CAD build for the part. Positions are in the model's coordinates, mm. A direction names the side the tool comes from. Give positions to 0.01 mm unless a question says otherwise; leave off trailing zeros. Loops run counter-clockwise (first coordinate to the right, second up) from the corner with the lowest first, then second, coordinate; pieces in that order, holes last.
Item 1: Mould opens along Z. For faces 4 (the flat face through (0, 0, -8)), 5 (the cylindrical face through (4.46, 0.59, -0.25)), 6 (the cylindrical face through (5, 1.6, 6.2)), 7 (the flat face through (0, 0, 9.76)) say: released by +Z, released by -Z, zero draft, split by the parting line, or undercut.
Item 2: Saw through at D-D on z = -2. Give the cut face in (x, y), plus the area to 3 significant figures.
Item 3: Which spindle directions (+Z, -Z, +X, -X, +Y, -Y) get a long thin tool onto all of the face, cutting with end or side? Do faces 1 (the cylindrical face through (-1.91, -8.62, 1.36)), 2 (the cylindrical face through (4.46, 0.59, -7.51)), 3 (the flat face through (4, -4, 2.76)). Say none if no direction does.
Item 4: Drop flat-ended pins along their axis: P1, Ø1, axis at x = 2.5, z = 0, coming from the +Y side; P2, Ø8, axis at y = -3.5, z = -5.5, coming from the -X side; P3, Ø4, axis at y = -4, z = 3, coming from the +X side. Give the stop position or say it passes through.
Item 5: Saw through at C-C on z = 1.5. Give the cut face in (x, y), plus the area to 3 significant figures.
Item 6: Probe probe 1 along Z at (x, y) = (4.5, -4.5); probe 2 along Z at (x, y) = (3, -4.25); probe 3 along X at (y, z) = (-1.5, -3). List the from-to ranges inside material, lowest first.
from build123d import *

# Parameters (mm, degrees)
F0_R     = 8.83
F1_DEPTH = 2.76
F4_R     = 5.25
F5_DEPTH = 7


with BuildPart() as f1:
    # F0 (on Top) → F1 (new body)
    with BuildSketch(Plane.XY):
        Circle(F0_R)
    extrude(amount=F1_DEPTH)

    # F2 (on Right) → F3 (revolve)
    with BuildSketch(Plane.YZ):
        Polygon((0, -8), (0, 0), (-4.5, 0), (-4.5, -0.5), (-5, -0.5), (-5, -0.666667), (-4.5, -2.666667), (-5, -2.666667), (-5, -2.833333), (-4.5, -4.833333), (-5, -4.833333), (-5, -5), (-4.5, -7), (-4.5, -8), align=None)
    revolve(axis=Axis((0, 0, -4), (0, 0, 1)))

    # F4 (on face) → F5 (join)
    with BuildSketch(Plane.XY.offset(2.76)):
        Circle(F4_R)
    extrude(amount=F5_DEPTH)


solid = f1.part
Results below:
1. face 4: released by -Z
1. face 5: undercut
1. face 6: zero draft
1. face 7: released by +Z
2. outline: circle Ø9.33 at (0, 0)
2. area: 68.4 mm2
3. face 1: +Z, -Z
3. face 2: -Z
3. face 3: +Z
4. P1: stops at y = 8.6
4. P2: stops at x = -5
4. P3: stops at x = 8.6
5. outline: circle Ø17.66 at (0, 0)
5. area: 245 mm2
6. probe 1: z = 0 to 2.76
6. probe 2: z = 0 to 9.76
6. probe 3: x = -4.73 to 4.73
